CAD build for the part. Positions are in the model's coordinates, mm. A direction names the side the tool comes from. Coordinates: 2 decimals unless noted, no trailing zeros. Loops run counter-clockwise (first coordinate to the right, second up) from the corner with the lowest first, then second, coordinate; pieces in that order, holes last. Notation, with made-up numbers: (-29, 71.25) -> (23, 71.25) arc R26 ccw to (23, 108.25) -> close; hole circle Ø6 at (81, -2). An arc over 180 degrees is marked (long way). Write item = value, one per line. Start each with the question number.
(1) Drill centre lines: line 1 (Y direction, x = 0.25, z = 22); line 2 (Y direction, x = 0, z = 7.75); line 3 (Z direction, x = 3.75, y = 8.5). Where is each one in solid material? Low to high. Write a range as from..to.
(2) Flat gauge pins, fed straight in: P1, Ø5, axis at x = 0, y = 7.5, coming from the +Z side; P2, Ø1.8, axis at x = -6.01, y = 6.01, coming from the -Z side; P3, Ø1.5, axis at x = 8.5, y = 4, coming from the -Z side; P4, Ø1.5, axis at y = 9.5, z = 14.5, coming from the +X side. Where does each tip first touch, or does it go through?
(3) Band-saw the part on B-B (y = 0). Write the cut outline in (x, z) (3 decimals).
(4) Pull direction Y, two halves, no side cores. Call faces 1 (the face through (-0.128, -11.463, 7.117)), 2 (the face through (0, 0, 0)), 3 (the face through (3.815, -6.299, 20.126)), 4 (the face through (2, 6, 11)): +Y half, -Y half, draft (parallel to the pull), parting line (faces both ways), or undercut.
(5) Band-saw the part on C-C (z = 13). Write the cut outline in (x, y).
(6) Band-saw the part on A-A (z = 16.75). Write the cut outline in (x, y), and give its area (3 significant figures).
(7) Tool access for faces 5 (the face through (0, 2.5, 22)), 6 (the face through (-0.867, 3.595, 20.126)), 7 (the face through (6, -6, 5)): list every direction of +Z, -Z, +X, -X, +Y, -Y with a clear straight run to the whole face (end or side of a thin tool).
(8) Band-saw the part on D-D (z = 4.5). Write the cut outline in (x, y), and give its area (3 significant figures).
```python
from build123d import *

# Parameters (mm, degrees)
F0_R      = 12.5
F1_DEPTH  = 29
F2_W      = 35.4545446894
F2_H      = 5
F3_DEPTH  = 15
F5_D      = 4
F4_R      = 4
F6_DEPTH  = 18
F9_D      = 2
F9_DEPTH  = 0.5
F9_START  = 0.0400643
F9_TIP    = 0.600860619
F10_R     = 0.025
F12_R     = 1.5
F13_DEPTH = 5


with BuildPart() as f1:
    # F0 (on Top) → F1 (new body)
    with BuildSketch(Plane.XY):
        Circle(F0_R)
    extrude(amount=F1_DEPTH)

    # F2 (on face) → F3 (cut)
    with BuildSketch(Plane.XY.offset(29)):
        with Locations((4.610654898, 0)):
            Rectangle(F2_W, F2_H)
    extrude(amount=-F3_DEPTH, mode=Mode.SUBTRACT)

    # F5 (through all)
    with Locations(Plane.XY.offset(29)):
        with Locations((0, 7.5), (0, -7.5)):
            Hole(F5_D / 2)

    # F4 (on face) → F6 (cut)
    with BuildSketch(Plane.XY.offset(29)):
        with Locations((0, 7.5)):
            Circle(F4_R)
        with Locations((0, -7.5)):
            Circle(F4_R)
    extrude(amount=-F6_DEPTH, mode=Mode.SUBTRACT)

    # F9
    # its depths count from where the whole tool has entered the part; down to there all is cleared
    with Locations(Plane.XZ.offset(12.5).offset(-F9_START)):
        with Locations((0, 7)):
            Hole(F9_D / 2, depth=F9_DEPTH)
            with Locations((0, 0, -(F9_DEPTH + F9_TIP / 2))):  # 118° drill point
                Cone(0, F9_D / 2, F9_TIP, mode=Mode.SUBTRACT)

    # F10 (on Front) → F11 (revolve, cut)
    with BuildSketch(Plane.XZ):
        with Locations((12.5041836873, 7)):
            Circle(F10_R)
    revolve(axis=Axis((0, 0, 4.1495896876), (0, 0, -1)), mode=Mode.SUBTRACT)

    # F12 (on face) → F13 (cut)
    with BuildSketch(Plane(origin=(0, 0, 0), x_dir=(1, 0, 0), z_dir=(0, 0, -1))):
        with Locations((6.0104076401, 6.0104076401)):
            Circle(F12_R)
        with Locations((-6.0104076401, -6.0104076401)):
            Circle(F12_R)
    extrude(amount=-F13_DEPTH, mode=Mode.SUBTRACT)


solid = f1.part
```
Findings below:
q1.line_1 = -12.5..-11.49, -3.51..-2.5, 2.5..3.51, 11.49..12.5
q1.line_2 = -11.81..-9.5, -5.5..5.5, 9.5..12.5
q1.line_3 = 0..11
q2.P1 = 11
q2.P2 = 5
q2.P3 = 0
q2.P4 = 8.93
q3.outline = (-12.5, 0) -> (12.5, 0) -> (12.5, 6.975) arc R0.025 cw to (12.5, 7.025) -> (12.5, 14) -> (-12.5, 14) -> (-12.5, 7.025) arc R0.025 cw to (-12.5, 6.975) -> close
q4.face_1 = -Y half
q4.face_2 = draft
q4.face_3 = undercut
q4.face_4 = undercut
q5.outline = circle Ø25 at (0, 0); hole circle Ø8 at (0, -7.5); hole circle Ø8 at (0, 7.5)
q6.outline = (-12.25, -2.5) arc R12.5 ccw to (12.25, -2.5) -> close; (-12.25, 2.5) -> (12.25, 2.5) arc R12.5 ccw to start; hole circle Ø8 at (0, -7.5); hole circle Ø8 at (0, 7.5)
q6.area = 266 mm²
q7.face_5 = +Z, +X, -X
q7.face_6 = +Z
q7.face_7 = -Z
q8.outline = circle Ø25 at (0, 0); hole circle Ø3 at (-6.01, 6.01); hole circle Ø4 at (0, -7.5); hole circle Ø4 at (0, 7.5); hole circle Ø3 at (6.01, -6.01)
q8.area = 452 mm²
